Build history of the part. All positions in model axes, mm. Round coordinates to 2 decimals unless told otherwise and drop trailing zeros. Write each loop counter-clockwise with the first axis right and the second up, starting at its lowest first coordinate (ties: lowest second). Pieces come first, ordered by that corner, then holes. Notation, with made-up numbers: (-22, 69.5) -> (8, 69.5) arc R23 ccw to (8, 90.5) -> close; hole circle Ø6 at (6, -40). An arc over 180 degrees is marked (long way). Answer in a Markdown table with one row per item. Add a question column.
from build123d import *

# Parameters (mm, degrees)
SKETCH1_R           = 82.55
SKETCH1_R_2         = 3.048
BOSS_EXTRUDE1_DEPTH = 5.08
SKETCH2_W           = 5.08
SKETCH2_H           = 5.08
CUT_EXTRUDE1_DEPTH  = 5.08


with BuildPart() as part:
    # Sketch1 → Boss-Extrude1 (new body)
    with BuildSketch(Plane(origin=(0, 0, 0), x_dir=(1, 0, 0), z_dir=(0, 1, 0))):
        with Locations(Location((-36.198285131, 29.074154547, 0), (0, 0, 270))):
            Circle(SKETCH1_R)
        with Locations(Location((-36.198285131, 29.074154547, 0), (0, 0, 270))):
            Circle(SKETCH1_R_2, mode=Mode.SUBTRACT)
        Polygon((-36.198285131, 96.384154547), (-33.658285131, 106.544154547), (-33.658285131, 81.144154547), (-36.198285131, 91.304154547), (-38.738285131, 81.144154547), (-38.738285131, 106.544154547), align=None, mode=Mode.SUBTRACT)
        Polygon((31.111714869, 29.074154547), (41.271714869, 26.534154547), (15.871714869, 26.534154547), (26.031714869, 29.074154547), (15.871714869, 31.614154547), (41.271714869, 31.614154547), align=None, mode=Mode.SUBTRACT)
        Polygon((-36.198285131, -38.235845453), (-38.738285131, -48.395845453), (-38.738285131, -22.995845453), (-36.198285131, -33.155845453), (-33.658285131, -22.995845453), (-33.658285131, -48.395845453), align=None, mode=Mode.SUBTRACT)
        Polygon((-103.508285131, 29.074154547), (-113.668285131, 31.614154547), (-88.268285131, 31.614154547), (-98.428285131, 29.074154547), (-88.268285131, 26.534154547), (-113.668285131, 26.534154547), align=None, mode=Mode.SUBTRACT)
    extrude(amount=BOSS_EXTRUDE1_DEPTH)

    # Sketch2 → Cut-Extrude1 (cut)
    with BuildSketch(Plane(origin=(0, 5.08, 0), x_dir=(1, 0, 0), z_dir=(0, 1, 0))):
        with Locations((-0.638285131, 22.724154547)):
            Rectangle(SKETCH2_W, SKETCH2_H)
        with Locations((-0.638285131, 45.584154547)):
            Rectangle(SKETCH2_W, SKETCH2_H)
        with Locations((-0.638285131, 35.424154547)):
            Rectangle(SKETCH2_W, SKETCH2_H)
        with Locations((-0.638285131, 12.564154547)):
            Rectangle(SKETCH2_W, SKETCH2_H)
        with Locations((-71.758285131, 12.564154547)):
            Rectangle(SKETCH2_W, SKETCH2_H)
        with Locations((-71.758285131, 22.724154547)):
            Rectangle(SKETCH2_W, SKETCH2_H)
        with Locations((-71.758285131, 35.424154547)):
            Rectangle(SKETCH2_W, SKETCH2_H)
        with Locations((-71.758285131, 45.584154547)):
            Rectangle(SKETCH2_W, SKETCH2_H)
    extrude(amount=-CUT_EXTRUDE1_DEPTH, mode=Mode.SUBTRACT)


solid = part.part
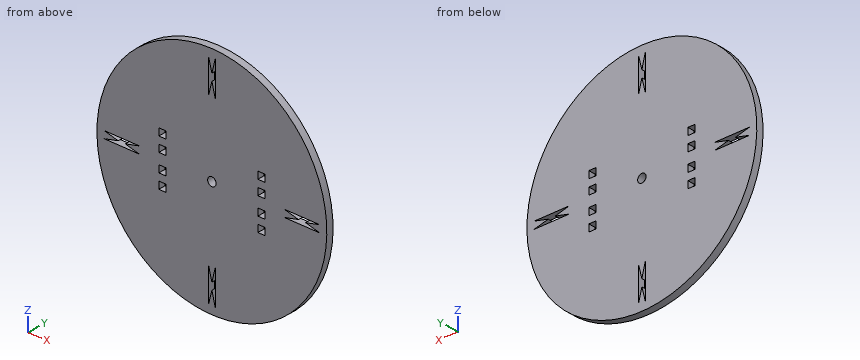
(1) Saw through at D-D (x = 0). List the corners of the cut face in (y, z), plus the area to 3 significant figures.
(2) Saw through at A-A (z = -87.5). List the corners of the cut face in (x, y), plus the area to 3 significant figures.
(3) Saw through at B-B (x = 34.5). List the corners of the cut face in (y, z).
(4) Saw through at C-C (y = 3.1). Count the separate pieces of the cut face and the enclosed holes in it, plus the area to 3 significant figures.
(5) Drop flat-ended pins along their axis: P1, Ø1.5, axis at x = -71, y = 3.5, coming from the -Z side; P2, Ø4, axis at x = -65, z = -82.5, coming from the -Y side; P3, Ø1.5, axis at y = 2.5, z = -46.5, coming from the -X side; P4, Ø2.5, axis at y = 2.5, z = -23, coming from the -X side. Give the stop position or say it passes through.
(6) Probe line 1 along X through (y, z) = (0.3, 39.5); line 2 along X through (y, z) = (1.95, 31); line 3 along Z through (x, y) = (-111.5, 2.4). List the from-to ranges inside material, lowest first.
Answer sheet:
| question | item | result |
|---|---|---|
| 1 | outline | (0, -103.26) -> (5.08, -103.26) -> (5.08, -48.12) -> (0, -48.12) -> close; (0, -43.04) -> (5.08, -43.04) -> (5.08, -37.96) -> (0, -37.96) -> close; (0, -32.88) -> (5.08, -32.88) -> (5.08, -25.26) -> (0, -25.26) -> close; (0, -20.18) -> (5.08, -20.18) -> (5.08, -15.1) -> (0, -15.1) -> close; (0, -10.02) -> (5.08, -10.02) -> (5.08, 45.12) -> (0, 45.12) -> close |
| 1 | area | 651 mm² |
| 2 | outline | (-94.52, 0) -> (-38.74, 0) -> (-38.74, 5.08) -> (-94.52, 5.08) -> close; (-37.15, 0) -> (-35.25, 0) -> (-35.25, 5.08) -> (-37.15, 5.08) -> close; (-33.66, 0) -> (22.12, 0) -> (22.12, 5.08) -> (-33.66, 5.08) -> close |
| 2 | area | 576 mm² |
| 3 | outline | (0, -71.69) -> (5.08, -71.69) -> (5.08, -31.61) -> (0, -31.61) -> close; (0, -29.92) -> (5.08, -29.92) -> (5.08, -28.23) -> (0, -28.23) -> close; (0, -26.53) -> (5.08, -26.53) -> (5.08, 13.54) -> (0, 13.54) -> close |
| 4 | separate pieces | 1 |
| 4 | enclosed holes | 13 |
| 4 | area | 20,900 mm² |
| 5 | P1 | stops at z = -104.27 |
| 5 | P2 | stops at y = 0 |
| 5 | P3 | stops at x = -117.05 |
| 5 | P4 | stops at x = -118.61 |
| 6 | line 1 | x = -82.16 to -38.74, -36.51 to -35.88, -33.66 to 9.76 |
| 6 | line 2 | x = -92.82 to -38.74, -36.74 to -35.66, -33.66 to 20.42 |
| 6 | line 3 | z = -62.9 to -31.61, -31.07 to -27.08, -26.53 to 4.75 |
